```python
from build123d import *

# Parameters (mm, degrees)
BASE_EXTRUDE_DEPTH              = 5
BOSS_EXTRUDE1_DEPTH             = 56.7
BOSS_EXTRUDE3_DEPTH             = 5
F_3_4_DIAMETER_HOLE1_D          = 3.4
F_4_40_TAPPED_HOLE1_D           = 2.2606
F_4_40_TAPPED_HOLE1_DEPTH       = 8.8646
F_4_40_TAPPED_HOLE1_CBORE_D     = 2.8448
F_4_40_TAPPED_HOLE1_CBORE_DEPTH = 5.6896
F_4_40_TAPPED_HOLE1_TIP         = 0.679152758
F_4_40_TAPPED_HOLE2_D           = 3.4544
F_4_40_TAPPED_HOLE2_CBORE_D     = 4.1656
F_4_40_TAPPED_HOLE2_CBORE_DEPTH = 8.3312
CUT_EXTRUDE1_DEPTH              = 2.54
HOLE1_D                         = 3.1877
HOLE1_DEPTH                     = 2.54
SKETCH14_W                      = 9.5
SKETCH14_H                      = 14.3
BOSS_EXTRUDE2_DEPTH             = 12.24


with BuildPart() as part:
    # Sketch1 → Base-Extrude (new body)
    with BuildSketch(Plane.XY.offset(-942.568622791)):
        Polygon((-5.8406, 18.9), (17.6094, 18.9), (17.6094, 3.98), (17.2294, 3.6), (17.2294, -3.6), (17.6094, -3.98), (17.6094, -18.9), (-5.8406, -18.9), align=None)
    extrude(amount=BASE_EXTRUDE_DEPTH)

    # Sketch3 → Boss-Extrude1 (add)
    with BuildSketch(Plane(origin=(0, 0, -942.568622791), x_dir=(-1, 0, 0), z_dir=(0, 0, -1))):
        Polygon((-17.6094, 3.98), (-17.6094, 18.9), (-7.3406, 18.9), (-7.3406, -18.9), (-17.6094, -18.9), (-17.6094, -3.98), (-17.2294, -3.6), (-17.2294, 3.6), align=None)
    extrude(amount=BOSS_EXTRUDE1_DEPTH)

    # Sketch15 → Boss-Extrude3 (add)
    with BuildSketch(Plane.XY.offset(-937.568622791)):
        Polygon((17.6094, -3.98), (17.2294, -3.6), (17.2294, 3.6), (17.6094, 3.98), align=None)
    extrude(amount=-BOSS_EXTRUDE3_DEPTH)

    # 3.4 Diameter Hole1 (through all)
    with Locations(Plane(origin=(17.2294, 0, 0), x_dir=(0, 0, -1), z_dir=(1, 0, 0))):
        with Locations((959.868622791, 0), (974.868622791, 0)):
            Hole(F_3_4_DIAMETER_HOLE1_D / 2)

    # #4-40 Tapped Hole1
    with Locations(Plane(origin=(17.6094, 0, 0), x_dir=(0, 0, -1), z_dir=(1, 0, 0))):
        with Locations((948.568622791, 11.5), (973.568622791, 11.5), (948.568622791, -11.5), (973.568622791, -11.5)):
            CounterBoreHole(F_4_40_TAPPED_HOLE1_D / 2, F_4_40_TAPPED_HOLE1_CBORE_D / 2, F_4_40_TAPPED_HOLE1_CBORE_DEPTH, depth=F_4_40_TAPPED_HOLE1_DEPTH)
            with Locations((0, 0, -(F_4_40_TAPPED_HOLE1_DEPTH + F_4_40_TAPPED_HOLE1_TIP / 2))):  # 118° drill point
                Cone(0, F_4_40_TAPPED_HOLE1_D / 2, F_4_40_TAPPED_HOLE1_TIP, mode=Mode.SUBTRACT)

    # #4-40 Tapped Hole2 (through all)
    with Locations(Plane.XY.offset(-937.568622791)):
        with Locations((4.6594, 16), (4.6594, -16)):
            CounterBoreHole(F_4_40_TAPPED_HOLE2_D / 2, F_4_40_TAPPED_HOLE2_CBORE_D / 2, F_4_40_TAPPED_HOLE2_CBORE_DEPTH)

    # Sketch11 → Cut-Extrude1 (cut)
    with BuildSketch(Plane(origin=(17.2294, 0, 0), x_dir=(0, 0, -1), z_dir=(1, 0, 0))):
        with BuildLine():
            Line((966.162472791, 1.59385), (966.974772791, 1.59385))
            ThreePointArc((966.974772791, 1.59385), (968.568622791, 0), (966.974772791, -1.59385))
            Line((966.974772791, -1.59385), (966.162472791, -1.59385))
            ThreePointArc((966.162472791, -1.59385), (964.568622791, 0), (966.162472791, 1.59385))
        make_face()
    extrude(amount=-CUT_EXTRUDE1_DEPTH, mode=Mode.SUBTRACT)

    # Hole1
    with Locations(Plane(origin=(17.2294, 0, 0), x_dir=(0, 0, -1), z_dir=(1, 0, 0))):
        with Locations((948.568622791, 0)):
            Hole(HOLE1_D / 2, depth=HOLE1_DEPTH)

    # Sketch14 → Boss-Extrude2 (add)
    with BuildSketch(Plane(origin=(0, 18.9, 0), x_dir=(-1, 0, 0), z_dir=(0, 1, 0))):
        with Locations((-12.8494, -977.918622791)):
            Rectangle(SKETCH14_W, SKETCH14_H)
    extrude(amount=BOSS_EXTRUDE2_DEPTH)


solid = part.part
```
Check sheet for the modelled part. Datum: model origin and axes. Units: mm. A direction names the side the tool comes from. Give positions to 0.01 mm unless a question says otherwise; leave off trailing zeros. Order: outer loops, then holes, each group sorted by start corner. A loop starts at its lowest first (then second) coordinate and runs counter-clockwise, first axis right, second up. Notation, with made-up numbers: M 83.25,21.5 L 116.25,21.5 A20 cw 116.25,40.5 Z; hole C 42.25,88 d9. An arc over 180 degrees is marked long. Answer in a Markdown table with one row per item.
1) Cross-section at C-C, the plane x = 10.5. Enter the section's corners in (y, z), plus the area to 3 significant figures.
Filled sheet:
| item | result |
|---|---|
| outline | M -18.9,-999.27 L 18.9,-999.27 L 18.9,-985.07 L 31.14,-985.07 L 31.14,-970.77 L 18.9,-970.77 L 18.9,-937.57 L -18.9,-937.57 Z; hole C -11.5,-973.57 d2.26; hole C -11.5,-948.57 d2.26; hole C 0,-974.87 d3.4; hole C 0,-959.87 d3.4; hole C 11.5,-973.57 d2.26; hole C 11.5,-948.57 d2.26 |
| area | 2,470 mm2 |
2) Cross-section at A-A, the plane y = 0. Enter the section's corners in (x, z), plus the area to 3 significant figures.
Filled sheet:
| item | result |
|---|---|
| outline | M -5.84,-942.57 L 7.34,-942.57 L 7.34,-958.17 L 17.23,-958.17 L 17.23,-950.16 L 14.69,-950.16 L 14.69,-946.97 L 17.23,-946.97 L 17.23,-942.57 L 17.61,-942.57 L 17.61,-937.57 L -5.84,-937.57 Z; M 7.34,-999.27 L 17.23,-999.27 L 17.23,-976.57 L 7.34,-976.57 Z; M 7.34,-973.17 L 17.23,-973.17 L 17.23,-968.57 L 14.69,-968.57 L 14.69,-964.57 L 17.23,-964.57 L 17.23,-961.57 L 7.34,-961.57 Z |
| area | 592 mm2 |
3) Access from +Z, -Z, +X, -X, +Y, -Y to the whole of each face (thin tool, end or side, straight path). Record for faces 1 (the flat face through (13, 31.14, -978)), 2 (the flat face through (8.099, 25, -978)), 3 (the cylindrical face through (15.98, -0.04, -964.57)).
Filled sheet:
| item | result |
|---|---|
| face 1 | +Z, -Z, +X, -X, +Y |
| face 2 | +Z, -Z, -X, +Y |
| face 3 | +X |
4) Cross-section at B-B, the plane y = 16. Enter the section's corners in (x, z), plus the area to 3 significant figures.
Filled sheet:
| item | result |
|---|---|
| outline | M -5.84,-942.57 L 2.58,-942.57 L 2.58,-937.57 L -5.84,-937.57 Z; M 6.74,-942.57 L 7.34,-942.57 L 7.34,-999.27 L 17.61,-999.27 L 17.61,-937.57 L 6.74,-937.57 Z |
| area | 679 mm2 |
5) Release check for a two-part mould opening along X. For faces 4 (the cylindrical face through (10.3, -11.5, -974.7)), 5 (the cylindrical face through (5.779, 17.756, -940.034)), 6 (the flat face through (7.341, 0, -971)) record: +X half, -X half, draft (parallel to the pull), parting line (faces both ways), or undercut.
Filled sheet:
| item | result |
|---|---|
| face 4 | draft |
| face 5 | undercut |
| face 6 | -X half |
6) Gauge pin test, flat ends, axial feed: P1, Ø4, axis at y = 8.5, z = -947, coming from the -X side; P2, Ø0.9, axis at x = 16, z = -966.5, coming from the +Y side; P3, Ø1.4, axis at y = 11.5, z = -973.57, coming from the +X side; P4, Ø2, axis at x = 6, z = -961, coming from the +Y side. Record the tip position at first contact, or that the pin passes through.
Filled sheet:
| item | result |
|---|---|
| P1 | stops at x = 7.34 |
| P2 | stops at y = 18.9 |
| P3 | stops at x = 8.49 |
| P4 | passes through |
7) Thickness scan on L1, parallel to Z at x = 10.05, y = -11.5; L2, parallel to Z at x = 14.25, y = -12.5; L3, parallel to Z at x = 5.5, y = -2.5. Record the ranges inside material, lowest first. Write a range as [from, to].
Filled sheet:
| item | result |
|---|---|
| L1 | z = [-999.27, -974.7], [-972.44, -949.7], [-947.44, -937.57] |
| L2 | z = [-999.27, -974.58], [-972.56, -949.58], [-947.56, -937.57] |
| L3 | z = [-942.57, -937.57] |
8) Cross-section at D-D, the plane x = 15.75. Count the separate pieces of the cut face and the enclosed holes in it, plus the area to 3 significant figures.
Filled sheet:
| item | result |
|---|---|
| separate pieces | 1 |
| enclosed holes | 8 |
| area | 2,450 mm2 |
